```python
from build123d import *

# Parameters (mm, degrees)
SKETCH_1_W      = 65
SKETCH_1_H      = 90
SKETCH_1_R      = 3.2
EXTRUDE_1_DEPTH = 5
FILLET_1_R      = 10
SKETCH_2_W      = 17.5
SKETCH_2_H      = 60
EXTRUDE_2_DEPTH = 55
FILLET_2_R      = 10
FILLET_3_R      = 1


with BuildPart() as part:
    # 스케치1 → 보스-돌출1 (new body)
    with BuildSketch(Plane(origin=(0, 0, 0), x_dir=(1, 0, 0), z_dir=(0, 1, 0))):
        with Locations((0, -12.5)):
            Rectangle(SKETCH_1_W, SKETCH_1_H)
        with Locations((-25, 25)):
            Circle(SKETCH_1_R, mode=Mode.SUBTRACT)
        with Locations((25, 25)):
            Circle(SKETCH_1_R, mode=Mode.SUBTRACT)
        with Locations((25, 0)):
            Circle(SKETCH_1_R, mode=Mode.SUBTRACT)
        with Locations((-25, 0)):
            Circle(SKETCH_1_R, mode=Mode.SUBTRACT)
        with Locations((25, -50)):
            Circle(SKETCH_1_R, mode=Mode.SUBTRACT)
        with Locations((-25, -50)):
            Circle(SKETCH_1_R, mode=Mode.SUBTRACT)
        with Locations((0, 25)):
            Circle(SKETCH_1_R, mode=Mode.SUBTRACT)
        with Locations((0, -50)):
            Circle(SKETCH_1_R, mode=Mode.SUBTRACT)
        with Locations((25, -25)):
            Circle(SKETCH_1_R, mode=Mode.SUBTRACT)
        with Locations((-25, -25)):
            Circle(SKETCH_1_R, mode=Mode.SUBTRACT)
    extrude(amount=EXTRUDE_1_DEPTH)

    # 필렛1
    fillet_1_edges = [part.edges().sort_by_distance(p)[0] for p in [
        (-32.5, 2.5, -32.5),
        (32.5, 2.5, -32.5),
        (32.5, 2.5, 57.5),
        (-32.5, 2.5, 57.5),
    ]]
    fillet(fillet_1_edges, radius=FILLET_1_R)

    # 스케치2 → 보스-돌출2 (add)
    with BuildSketch(Plane(origin=(0, 5, 0), x_dir=(1, 0, 0), z_dir=(0, 1, 0))):
        with Locations((0, -12.5)):
            Rectangle(SKETCH_2_W, SKETCH_2_H)
    extrude(amount=EXTRUDE_2_DEPTH)

    # 필렛2
    fillet_2_edges = [part.edges().sort_by_distance(p)[0] for p in [
        (8.75, 32.5, 42.5),
        (8.75, 32.5, -17.5),
        (0, 60, -17.5),
        (0, 60, 42.5),
        (8.75, 60, 12.5),
    ]]
    fillet(fillet_2_edges, radius=FILLET_2_R)

    # 필렛3
    fillet_3_edges = [part.edges().sort_by_distance(p)[0] for p in [
        (-8.75, 57.071067812, -14.571067812),
        (5.821067812, 5, -14.571067812),
        (5.821067812, 5, 39.571067812),
        (-8.75, 5, 12.5),
        (-5, 5, 42.5),
        (-8.75, 60, 12.5),
        (8.75, 5, 12.5),
        (-5, 5, -17.5),
        (-8.75, 27.5, -17.5),
        (-8.75, 27.5, 42.5),
        (-8.75, 57.071067812, 39.571067812),
    ]]
    fillet(fillet_3_edges, radius=FILLET_3_R)


solid = part.part
```
Model file for the job. Use its own axes, mm. A direction names the side the tool comes from. Give positions to 0.01 mm unless a question says otherwise; leave off trailing zeros. Loops run counter-clockwise (first coordinate to the right, second up) from the corner with the lowest first, then second, coordinate; pieces in that order, holes last. Notation, with made-up numbers: M 40.25,-3 L 86.25,-3 A25 cw 86.25,24 Z; hole C 7.25,76.5 d10. An arc over 180 degrees is marked long. Use one line per item in the form item = value.
Item 1: Flat gauge pins, fed straight in: pin 1 Ø5 at (x, z) = (-23, -12.5) entering from +Y; pin 2 Ø5 at (x, z) = (2, 30.5) entering from +Y; pin 3 Ø1 at (x, z) = (-10.5, 30.5) entering from -Y; pin 4 Ø8 at (x, y) = (5, 19.5) entering from -Z. Where does each tip first touch, or does it go through?
Filled in:
pin_1 = 5
pin_2 = 59.97
pin_3 = 0
pin_4 = -17.24
Item 2: Two-plate mould, pull along X, no slides. Class faces 6 (the cylindrical face through (-29.65, 2.54, 54.49)), 7 (the flat face through (8.75, 28, 13)), 8 (the cylindrical face through (21.8, 2.5, -25.1)): released by +X, released by -X, zero draft, split by the parting line, or undercut.
Filled in:
face_6 = released by -X
face_7 = released by +X
face_8 = undercut
Item 3: Which spindle directions (+Z, -Z, +X, -X, +Y, -Y) get a long thin tool onto all of the face, cutting with end or side? Do faces 1 (the cylindrical face through (5.9, 28.31, -14.49)), 2 (the cylindrical face through (-28.2, 2.5, -0.1)), 3 (the flat face through (-5, 28, -17.5)), 4 (the flat face through (-8.75, 32, 13)), 5 (the flat face through (32.5, 2, 13)). Say none if no direction does.
Filled in:
face_1 = -Z, +X, +Y
face_2 = +Y, -Y
face_3 = -Z, +X, -X, +Y
face_4 = +Z, -Z, -X, +Y
face_5 = +Z, -Z, +X, +Y, -Y
Item 4: Slice it at D-D on y = 33. List the corners of the cut face in (x, z), and give its area (3 significant figures).
Filled in:
outline = M -8.75,-16.5 A1 ccw -7.75,-17.5 L -1.25,-17.5 A10 ccw 8.75,-7.5 L 8.75,32.5 A10 ccw -1.25,42.5 L -7.75,42.5 A1 ccw -8.75,41.5 Z
area = 1,010 mm^2
Item 5: Drill centre lines: L1, parallel to Z at x = -25, y = 2; L2, parallel to X at y = 3.5, z = -25.5; L3, parallel to X at y = 44, z = 1. Where is each one in solid material? Low to high.
Filled in:
L1 = -32.18 to -28.2, -21.8 to -3.2, 3.2 to 21.8, 28.2 to 46.8, 53.2 to 57.18
L2 = -32.04 to -28.16, -21.84 to -3.16, 3.16 to 21.84, 28.16 to 32.04
L3 = -8.75 to 8.75
Item 6: Slice it at A-A on z = 0. List the corners of the cut face in (x, y).
Filled in:
outline = M -32.5,0 L -28.2,0 L -28.2,5 L -32.5,5 Z; M -21.8,0 L 21.8,0 L 21.8,5 L 9.75,5 A1 cw 8.75,6 L 8.75,50 A10 ccw -1.25,60 L -7.75,60 A1 ccw -8.75,59 L -8.75,6 A1 cw -9.75,5 L -21.8,5 Z; M 28.2,0 L 32.5,0 L 32.5,5 L 28.2,5 Z
Item 7: Slice it at C-C on z = 50. List the corners of the cut face in (x, y).
Filled in:
outline = M -32.18,0 L -28.2,0 L -28.2,5 L -32.18,5 Z; M -21.8,0 L -3.2,0 L -3.2,5 L -21.8,5 Z; M 3.2,0 L 21.8,0 L 21.8,5 L 3.2,5 Z; M 28.2,0 L 32.18,0 L 32.18,5 L 28.2,5 Z
Item 8: Slice it at B-B on x = -25. List the corners of the cut face in (y, z), and give its area (3 significant figures).
Filled in:
outline = M 0,-32.18 L 5,-32.18 L 5,-28.2 L 0,-28.2 Z; M 0,-21.8 L 5,-21.8 L 5,-3.2 L 0,-3.2 Z; M 0,3.2 L 5,3.2 L 5,21.8 L 0,21.8 Z; M 0,28.2 L 5,28.2 L 5,46.8 L 0,46.8 Z; M 0,53.2 L 5,53.2 L 5,57.18 L 0,57.18 Z
area = 319 mm^2
